Design review of the part built by this model. Coordinates are the model's own, in mm. A direction names the side the tool comes from. Round coordinates to 2 decimals unless told otherwise and drop trailing zeros. Order: outer loops, then holes, each group sorted by start corner. A loop starts at its lowest first (then second) coordinate and runs counter-clockwise, first axis right, second up. Notation, with made-up numbers: M 9,18 L 28,18 A12 cw 28,31 Z; hole C 48.25,85 d1. An arc over 180 degrees is marked long. Write each question's results on one line, items separated by ' | '. Start each with the question number.
Item 1: The part is to be moulded in two halves that separate along Y. For faces 1 (the flat face through (3, -1.99, -48)), 2 (the flat face through (3, 6, 3.569)), 3 (the cylindrical face through (3, 0, -6)), say which applies: +Y half, -Y half, draft (parallel to the pull), parting line (faces both ways), or undercut.
Item 2: Machinability: for faces 4 (the cylindrical face through (2.958, -7.415, -1.127)), 5 (the flat face through (3, 1.99, -49)), which of the approach directions +Z, -Z, +X, -X, +Y, -Y give a long, thin tool a straight path to every point of the face, cutting with its end or side? Answer none if there is none.
Item 3: Take a section at A-A, the plane z = 0. Write out the cut boundary in (x, y).
Item 4: Take a section at D-D, the plane y = 0. Write out the cut boundary in (x, z).
Item 5: Take a section at B-B, the plane x = 3.5. Write out the cut boundary in (y, z).
Item 6: Take a section at C-C, the plane z = -70. Write out the cut boundary in (x, y).
Item 7: Wall thickness on line 1 (Y direction, x = 4.25, z = 0); line 2 (Y direction, x = 5.4, z = -76); line 3 (Z direction, x = 4.4, y = 5.25): over which ranges is each line inside the solid? List them lowest first. Write a range as [from, to].
Item 8: Clearance check with flat-ended pins moving along their axes: pin 1 (3 mm diameter, centred on x = 3.5, z = -54, fed in from +Y); pin 2 (1 mm diameter, centred on y = -4, z = -67.5, fed in from -X). State where each tip first meets the part, or that it passes through.
```python
from build123d import *

# Parameters (mm, degrees)
BOSS_EXTRUDE1_DEPTH = 6
FILLET1_R           = 10


with BuildPart() as part:
    # Sketch1 → Boss-Extrude1 (new body)
    with BuildSketch(Plane(origin=(0, 0, 0), x_dir=(0, 0, -1), z_dir=(1, 0, 0))):
        with BuildLine():
            ThreePointArc((7.23115504, 1.990074568), (2.942582115, 6.898638307), (-3.56853515, 6.596632238))
            Line((-3.56853515, 6.596632238), (-3.56853515, 4.823438285))
            ThreePointArc((-3.56853515, 4.823438285), (6, 0), (-3.56853515, -4.823438285))
            Line((-3.56853515, -4.823438285), (-3.56853515, -6.596632238))
            ThreePointArc((-3.56853515, -6.596632238), (2.942582115, -6.898638307), (7.23115504, -1.990074568))
            Line((7.23115504, -1.990074568), (85, -1.990074568))
            Line((85, -1.990074568), (85, 1.990074568))
            Line((85, 1.990074568), (7.23115504, 1.990074568))
        make_face()
    extrude(amount=BOSS_EXTRUDE1_DEPTH)

    # Fillet1
    fillet1_edges = [part.edges().sort_by_distance(p)[0] for p in [
        (3, 1.990074568, -7.23115504),
        (3, -1.990074568, -7.23115504),
    ]]
    fillet(fillet1_edges, radius=FILLET1_R)


solid = part.part
```
Results list:
1) face 1: -Y half | face 2: draft | face 3: undercut
2) face 4: +X, -X, -Y | face 5: -Z, +X, -X, +Y
3) outline: M 0,-7.5 L 6,-7.5 L 6,-6 L 0,-6 Z; M 0,6 L 6,6 L 6,7.5 L 0,7.5 Z
4) outline: M 0,-85 L 6,-85 L 6,-6 L 0,-6 Z
5) outline: M -6.6,3.57 A7.5 ccw -5.14,-5.46 A10 cw -1.99,-12.75 L -1.99,-85 L 1.99,-85 L 1.99,-12.75 A10 cw 5.14,-5.46 A7.5 ccw 6.6,3.57 L 4.82,3.57 A6 cw long -4.82,3.57 Z
6) outline: M 0,-1.99 L 6,-1.99 L 6,1.99 L 0,1.99 Z
7) line 1: [-7.5, -6], [6, 7.5] | line 2: [-1.99, 1.99] | line 3: [-5.36, -2.9], [2.9, 3.57]
8) pin 1: y = 1.99 | pin 2: through
